from build123d import *

# Parameters (mm, degrees)
SKETCH_1_W          = 152
SKETCH_1_H          = 60
EXTRUDE_1_DEPTH     = 3
FILLET_1_R          = 5
CUT_EXTRUDE_1_REACH = 83.762
SKETCH_2_R          = 1.525
CUT_EXTRUDE_2_REACH = 83.762
SKETCH_3_W          = 16
SKETCH_3_H          = 9
CUT_EXTRUDE_3_REACH = 83.762
SKETCH_4_R          = 1.525
CUT_EXTRUDE_4_REACH = 83.762
SKETCH_5_R          = 5.5


with BuildPart() as part:
    # 草图1 → 凸台-拉伸1 (new body)
    with BuildSketch(Plane(origin=(0, 0, 0), x_dir=(1, 0, 0), z_dir=(0, 1, 0))):
        Rectangle(SKETCH_1_W, SKETCH_1_H)
    extrude(amount=EXTRUDE_1_DEPTH)

    # 圆角1
    fillet_1_edges = [part.edges().sort_by_distance(p)[0] for p in [
        (76, 1.5, 30),
        (-76, 1.5, 30),
        (-76, 1.5, -30),
        (76, 1.5, -30),
    ]]
    fillet(fillet_1_edges, radius=FILLET_1_R)

    # 草图2 → 切除-拉伸1 (cut, up to next)
    with BuildSketch(Plane(origin=(0, 3, 0), x_dir=(1, 0, 0), z_dir=(0, 1, 0)), mode=Mode.PRIVATE) as cut_extrude_1_sk1:
        with Locations(Location((-66, -24, 0), (0, 0, 270))):
            Circle(SKETCH_2_R)
    cut_extrude_1_tool1 = extrude(cut_extrude_1_sk1.sketch, amount=-CUT_EXTRUDE_1_REACH, mode=Mode.PRIVATE) & part.part
    # 草图2 → 切除-拉伸1 (cut, up to next)
    with BuildSketch(Plane(origin=(0, 3, 0), x_dir=(1, 0, 0), z_dir=(0, 1, 0)), mode=Mode.PRIVATE) as cut_extrude_1_sk2:
        with Locations(Location((66, -24, 0), (0, 0, 270))):
            Circle(SKETCH_2_R)
    cut_extrude_1_tool2 = extrude(cut_extrude_1_sk2.sketch, amount=-CUT_EXTRUDE_1_REACH, mode=Mode.PRIVATE) & part.part
    # 草图2 → 切除-拉伸1 (cut, up to next)
    with BuildSketch(Plane(origin=(0, 3, 0), x_dir=(1, 0, 0), z_dir=(0, 1, 0)), mode=Mode.PRIVATE) as cut_extrude_1_sk3:
        with Locations(Location((66, 24, 0), (0, 0, 270))):
            Circle(SKETCH_2_R)
    cut_extrude_1_tool3 = extrude(cut_extrude_1_sk3.sketch, amount=-CUT_EXTRUDE_1_REACH, mode=Mode.PRIVATE) & part.part
    # 草图2 → 切除-拉伸1 (cut, up to next)
    with BuildSketch(Plane(origin=(0, 3, 0), x_dir=(1, 0, 0), z_dir=(0, 1, 0)), mode=Mode.PRIVATE) as cut_extrude_1_sk4:
        with Locations(Location((-66, 24, 0), (0, 0, 270))):
            Circle(SKETCH_2_R)
    cut_extrude_1_tool4 = extrude(cut_extrude_1_sk4.sketch, amount=-CUT_EXTRUDE_1_REACH, mode=Mode.PRIVATE) & part.part
    add(cut_extrude_1_tool1.solids().sort_by_distance((-66, 3, 24))[0], mode=Mode.SUBTRACT)
    add(cut_extrude_1_tool2.solids().sort_by_distance((66, 3, 24))[0], mode=Mode.SUBTRACT)
    add(cut_extrude_1_tool3.solids().sort_by_distance((66, 3, -24))[0], mode=Mode.SUBTRACT)
    add(cut_extrude_1_tool4.solids().sort_by_distance((-66, 3, -24))[0], mode=Mode.SUBTRACT)

    # 草图3 → 切除-拉伸2 (cut, up to next)
    with BuildSketch(Plane(origin=(0, 3, 0), x_dir=(1, 0, 0), z_dir=(0, 1, 0)), mode=Mode.PRIVATE) as cut_extrude_2_sk1:
        with BuildLine():
            Line((-8, -30), (-8, -21))
            ThreePointArc((-8, -21), (-11.354101966, -22.291900756), (-12.974937186, -25.5))
            ThreePointArc((-12.974937186, -25.5), (-14.595772405, -28.708099244), (-17.949874371, -30))
            Line((-17.949874371, -30), (-8, -30))
        make_face()
    cut_extrude_2_tool1 = extrude(cut_extrude_2_sk1.sketch, amount=-CUT_EXTRUDE_2_REACH, mode=Mode.PRIVATE) & part.part
    # 草图3 → 切除-拉伸2 (cut, up to next)
    with BuildSketch(Plane(origin=(0, 3, 0), x_dir=(1, 0, 0), z_dir=(0, 1, 0)), mode=Mode.PRIVATE) as cut_extrude_2_sk2:
        with Locations((0, -25.5)):
            Rectangle(SKETCH_3_W, SKETCH_3_H)
    cut_extrude_2_tool2 = extrude(cut_extrude_2_sk2.sketch, amount=-CUT_EXTRUDE_2_REACH, mode=Mode.PRIVATE) & part.part
    # 草图3 → 切除-拉伸2 (cut, up to next)
    with BuildSketch(Plane(origin=(0, 3, 0), x_dir=(1, 0, 0), z_dir=(0, 1, 0)), mode=Mode.PRIVATE) as cut_extrude_2_sk3:
        with BuildLine():
            ThreePointArc((12.974937186, -25.5), (11.354101966, -22.291900756), (8, -21))
            Line((8, -21), (8, -30))
            Line((8, -30), (17.949874371, -30))
            ThreePointArc((17.949874371, -30), (14.595772405, -28.708099244), (12.974937186, -25.5))
        make_face()
    cut_extrude_2_tool3 = extrude(cut_extrude_2_sk3.sketch, amount=-CUT_EXTRUDE_2_REACH, mode=Mode.PRIVATE) & part.part
    # 草图3 → 切除-拉伸2 (cut, up to next)
    with BuildSketch(Plane(origin=(0, 3, 0), x_dir=(1, 0, 0), z_dir=(0, 1, 0)), mode=Mode.PRIVATE) as cut_extrude_2_sk4:
        with BuildLine():
            ThreePointArc((-12.974937186, 25.5), (-11.354101966, 22.291900756), (-8, 21))
            Line((-8, 21), (-8, 30))
            Line((-8, 30), (-17.949874371, 30))
            ThreePointArc((-17.949874371, 30), (-14.595772405, 28.708099244), (-12.974937186, 25.5))
        make_face()
    cut_extrude_2_tool4 = extrude(cut_extrude_2_sk4.sketch, amount=-CUT_EXTRUDE_2_REACH, mode=Mode.PRIVATE) & part.part
    # 草图3 → 切除-拉伸2 (cut, up to next)
    with BuildSketch(Plane(origin=(0, 3, 0), x_dir=(1, 0, 0), z_dir=(0, 1, 0)), mode=Mode.PRIVATE) as cut_extrude_2_sk5:
        with Locations((0, 25.5)):
            Rectangle(SKETCH_3_W, SKETCH_3_H)
    cut_extrude_2_tool5 = extrude(cut_extrude_2_sk5.sketch, amount=-CUT_EXTRUDE_2_REACH, mode=Mode.PRIVATE) & part.part
    # 草图3 → 切除-拉伸2 (cut, up to next)
    with BuildSketch(Plane(origin=(0, 3, 0), x_dir=(1, 0, 0), z_dir=(0, 1, 0)), mode=Mode.PRIVATE) as cut_extrude_2_sk6:
        with BuildLine():
            Line((8, 30), (8, 21))
            ThreePointArc((8, 21), (11.354101966, 22.291900756), (12.974937186, 25.5))
            ThreePointArc((12.974937186, 25.5), (14.595772405, 28.708099244), (17.949874371, 30))
            Line((17.949874371, 30), (8, 30))
        make_face()
    cut_extrude_2_tool6 = extrude(cut_extrude_2_sk6.sketch, amount=-CUT_EXTRUDE_2_REACH, mode=Mode.PRIVATE) & part.part
    add(cut_extrude_2_tool1.solids().sort_by_distance((-10.749177, 3, 26.299455))[0], mode=Mode.SUBTRACT)
    add(cut_extrude_2_tool2.solids().sort_by_distance((0, 3, 25.5))[0], mode=Mode.SUBTRACT)
    add(cut_extrude_2_tool3.solids().sort_by_distance((10.749177, 3, 26.299455))[0], mode=Mode.SUBTRACT)
    add(cut_extrude_2_tool4.solids().sort_by_distance((-10.749177, 3, -26.299455))[0], mode=Mode.SUBTRACT)
    add(cut_extrude_2_tool5.solids().sort_by_distance((0, 3, -25.5))[0], mode=Mode.SUBTRACT)
    add(cut_extrude_2_tool6.solids().sort_by_distance((10.749177, 3, -26.299455))[0], mode=Mode.SUBTRACT)

    # 草图4 → 切除-拉伸3 (cut, up to next)
    with BuildSketch(Plane(origin=(0, 3, 0), x_dir=(1, 0, 0), z_dir=(0, 1, 0)), mode=Mode.PRIVATE) as cut_extrude_3_sk1:
        with Locations(Location((-47, -17, 0), (0, 0, 270))):
            Circle(SKETCH_4_R)
    cut_extrude_3_tool1 = extrude(cut_extrude_3_sk1.sketch, amount=-CUT_EXTRUDE_3_REACH, mode=Mode.PRIVATE) & part.part
    # 草图4 → 切除-拉伸3 (cut, up to next)
    with BuildSketch(Plane(origin=(0, 3, 0), x_dir=(1, 0, 0), z_dir=(0, 1, 0)), mode=Mode.PRIVATE) as cut_extrude_3_sk2:
        with Locations(Location((-47, 17, 0), (0, 0, 270))):
            Circle(SKETCH_4_R)
    cut_extrude_3_tool2 = extrude(cut_extrude_3_sk2.sketch, amount=-CUT_EXTRUDE_3_REACH, mode=Mode.PRIVATE) & part.part
    # 草图4 → 切除-拉伸3 (cut, up to next)
    with BuildSketch(Plane(origin=(0, 3, 0), x_dir=(1, 0, 0), z_dir=(0, 1, 0)), mode=Mode.PRIVATE) as cut_extrude_3_sk3:
        with Locations(Location((47, -17, 0), (0, 0, 270))):
            Circle(SKETCH_4_R)
    cut_extrude_3_tool3 = extrude(cut_extrude_3_sk3.sketch, amount=-CUT_EXTRUDE_3_REACH, mode=Mode.PRIVATE) & part.part
    # 草图4 → 切除-拉伸3 (cut, up to next)
    with BuildSketch(Plane(origin=(0, 3, 0), x_dir=(1, 0, 0), z_dir=(0, 1, 0)), mode=Mode.PRIVATE) as cut_extrude_3_sk4:
        with Locations(Location((47, 17, 0), (0, 0, 270))):
            Circle(SKETCH_4_R)
    cut_extrude_3_tool4 = extrude(cut_extrude_3_sk4.sketch, amount=-CUT_EXTRUDE_3_REACH, mode=Mode.PRIVATE) & part.part
    add(cut_extrude_3_tool1.solids().sort_by_distance((-47, 3, 17))[0], mode=Mode.SUBTRACT)
    add(cut_extrude_3_tool2.solids().sort_by_distance((-47, 3, -17))[0], mode=Mode.SUBTRACT)
    add(cut_extrude_3_tool3.solids().sort_by_distance((47, 3, 17))[0], mode=Mode.SUBTRACT)
    add(cut_extrude_3_tool4.solids().sort_by_distance((47, 3, -17))[0], mode=Mode.SUBTRACT)

    # 草图5 → 切除-拉伸4 (cut, up to next)
    with BuildSketch(Plane(origin=(0, 3, 0), x_dir=(1, 0, 0), z_dir=(0, 1, 0)), mode=Mode.PRIVATE) as cut_extrude_4_sk1:
        with Locations(Location((-67, 12, 0), (0, 0, 270))):
            Circle(SKETCH_5_R)
    cut_extrude_4_tool1 = extrude(cut_extrude_4_sk1.sketch, amount=-CUT_EXTRUDE_4_REACH, mode=Mode.PRIVATE) & part.part
    # 草图5 → 切除-拉伸4 (cut, up to next)
    with BuildSketch(Plane(origin=(0, 3, 0), x_dir=(1, 0, 0), z_dir=(0, 1, 0)), mode=Mode.PRIVATE) as cut_extrude_4_sk2:
        with Locations(Location((67, -12, 0), (0, 0, 270))):
            Circle(SKETCH_5_R)
    cut_extrude_4_tool2 = extrude(cut_extrude_4_sk2.sketch, amount=-CUT_EXTRUDE_4_REACH, mode=Mode.PRIVATE) & part.part
    add(cut_extrude_4_tool1.solids().sort_by_distance((-67, 3, -12))[0], mode=Mode.SUBTRACT)
    add(cut_extrude_4_tool2.solids().sort_by_distance((67, 3, 12))[0], mode=Mode.SUBTRACT)


solid = part.part
Here's how the part is built. I have some questions about the finished solid (model axes, mm). Give positions to 0.01 mm unless a question says otherwise; leave off trailing zeros. Loops run counter-clockwise (first coordinate to the right, second up) from the corner with the lowest first, then second, coordinate; pieces in that order, holes last. Notation, with made-up numbers: (47.25, 53) -> (93.25, 53) arc R23 ccw to (93.25, 80) -> close; hole circle Ø11 at (71.25, 40). An arc over 180 degrees is marked (long way). One line per item, written item: value.
Q1. Suppose I cut it at A-A on z = -12. Please give me the cut outline in (x, y), then the cut area to 3 significant figures.
Answers follow:
outline: (-76, 0) -> (-72.5, 0) -> (-72.5, 3) -> (-76, 3) -> close; (-61.5, 0) -> (76, 0) -> (76, 3) -> (-61.5, 3) -> close
area: 423 mm^2
Q2. If I drill on line 1 along X through (y, z) = (1.3, -24) (3 decimals); line 2 along Z through (x, y) = (-66, 1.9) (3 decimals); line 3 along X through (y, z) = (1.4, 17) (3 decimals), over which ranges is the centre line in solid material (lowest first)?
Answers follow:
line 1: -76 to -67.525, -64.475 to -12.583, 12.583 to 64.475, 67.525 to 76
line 2: -30 to -25.525, -22.475 to -17.408, -6.592 to 22.475, 25.525 to 30
line 3: -76 to -48.525, -45.475 to 45.475, 48.525 to 64.709, 69.291 to 76
Q3. We'd pull the mould along Z, two halves only. Please class faces 1 (the face through (-45.7, 1.5, 17.8)), 2 (the face through (-45, 1, -30)), 3 (the face through (72.453, 1.521, 11.284)), 4 (the face through (44, 1, 30)): pulls with the +Z half, pulls with the -Z half, needs draft (parallel to the pull), parting line crosses it, or undercut.
Answers follow:
face 1: undercut
face 2: pulls with the -Z half
face 3: undercut
face 4: pulls with the +Z half
Q4. I'm going to push flat-ended pins straight in: pin 1 Ø4 at (x, z) = (47, -17) entering from -Y; pin 2 Ø1 at (x, y) = (4, 1.5) entering from +Z. Where does each tip first touch, or does it pass through?
Answers follow:
pin 1: y = 0
pin 2: z = 21
Q5. Suppose I cut it at B-B on x = 47. Please give me the cut outline in (y, z) (3 decimals).
Answers follow:
outline: (0, -30) -> (3, -30) -> (3, -18.525) -> (0, -18.525) -> close; (0, -15.475) -> (3, -15.475) -> (3, 15.475) -> (0, 15.475) -> close; (0, 18.525) -> (3, 18.525) -> (3, 30) -> (0, 30) -> close
Q6. Suppose I cut it at C-C on y = 1.2. State how many separate pieces and enclosed holes the cut face has, then the cut area to 3 significant figures.
Answers follow:
separate pieces: 1
enclosed holes: 10
area: 8,380 mm^2
Q7. Suppose I cut it at D-D on z = 10.5. Please give me the cut outline in (x, y).
Answers follow:
outline: (-76, 0) -> (61.71, 0) -> (61.71, 3) -> (-76, 3) -> close; (72.29, 0) -> (76, 0) -> (76, 3) -> (72.29, 3) -> close
